Check sheet for the modelled part. Datum: model origin and axes. Units: mm. Give positions to 0.01 mm unless a question says otherwise; leave off trailing zeros. Order: outer loops, then holes, each group sorted by start corner. A loop starts at its lowest first (then second) coordinate and runs counter-clockwise, first axis right, second up.
Item 1: Sectioned sample at A-A on y = 26. Record the boundary of the cut face in (x, z).
Item 2: Sectioned sample at B-B on y = 21.5. Count the separate pieces of the cut face and the enclosed holes in it, and give its area (3 significant figures).
Item 3: Material ranges on line 1 along Y through (x, z) = (22.5, 1.5); line 2 along Z through (x, y) = (20.5, 20); line 3 along X through (y, z) = (-3, 3.5), recorded low to high.
Item 4: Gauge pin test, flat ends, axial feed: P1, Ø5, axis at x = -7, z = 54.5, coming from the -Y side; P2, Ø5, axis at x = 13, y = -1, coming from the +Z side; P3, Ø10, axis at x = 26, z = 17.5, coming from the +Y side; P4, Ø5, axis at x = 29.75, z = 2.76, coming from the -Y side. Record the tip position at first contact, or that the pin passes through.
from build123d import *
from build123d.topology import SkipClean

# Parameters (mm, degrees)
BOSS_EXTRUDE1_START       = -4.7
BOSS_EXTRUDE1_DEPTH       = 4.7
BOSS_EXTRUDE2_OUTLINE_R   = 0.75
BOSS_EXTRUDE2_OUTLINE_R_2 = 2.5
BOSS_EXTRUDE2_DEPTH       = 0.3
SKETCH1_9_R               = 3.95
CUT_EXTRUDE2_DEPTH        = 0.7
SKETCH6_R                 = 0.75
SKETCH6_R_2               = 3.95
BOSS_EXTRUDE6_DEPTH       = 6.25
BOSS_EXTRUDE3_START       = 6.25
SKETCH2_R                 = 5.95
SKETCH2_R_2               = 4.2
BOSS_EXTRUDE3_DEPTH       = 16.25
SKETCH4_R                 = 5.95
SKETCH4_R_2               = 4.2
BOSS_EXTRUDE5_DEPTH       = 5
REVOLVE1_ANGLE            = 10
CUT_EXTRUDE3_DEPTH        = 79.445410831
CIRPATTERN1_COUNT         = 11
CIRPATTERN1_ANGLE         = 85
CUT_EXTRUDE4_DEPTH        = 79.445410831
LPATTERN1_COUNT           = 9
LPATTERN1_PITCH           = 3


# Read off the part's stored shape, not the designer's step: Boss-Extrude2
with BuildPart() as part:
    # Sketch1 → Boss-Extrude1 (new body)
    with BuildSketch(Plane.XZ.offset(-23.543068193).offset(BOSS_EXTRUDE1_START)):
        with BuildLine():
            Line((-0.472592015, 60.640230135), (-2.578285997, 64.210446846))
            ThreePointArc((-2.578285997, 64.210446846), (-11.633365316, 40.543634759), (0.19757138, 18.135123145))
            Line((0.19757138, 18.135123145), (26.104084692, -1.947430003))
            ThreePointArc((26.104084692, -1.947430003), (34.902992649, -0.218708783), (31.996731648, 8.264386483))
            Line((31.996731648, 8.264386483), (8.919209653, 17.677874535))
            ThreePointArc((8.919209653, 17.677874535), (-7.073200942, 36.689574632), (-0.472592015, 60.640230135))
        make_face()
        with BuildLine():
            ThreePointArc((14.223692018, 9.302922077), (13.639231125, 12.051374585), (16.311289521, 12.920678706))
            Line((16.311289521, 12.920678706), (30.419933466, 6.647779521))
            ThreePointArc((30.419933466, 6.647779521), (32.770289273, 5.300105007), (33.699453705, 2.75509961))
            ThreePointArc((33.699453705, 2.75509961), (31.093930231, -0.959046708), (26.714702885, 0.226703387))
            Line((26.714702885, 0.226703387), (14.223692018, 9.302922077))
        make_face(mode=Mode.SUBTRACT)
    extrude(amount=BOSS_EXTRUDE1_DEPTH)

    # Boss-Extrude2 outline → Boss-Extrude2 (add)
    with BuildSketch(Plane.XZ.offset(-23.543068193)):
        with BuildLine():
            Line((-0.472592015, 60.640230135), (-2.578285997, 64.210446846))
            ThreePointArc((-2.578285997, 64.210446846), (-11.633365316, 40.543634759), (0.19757138, 18.135123145))
            Line((0.19757138, 18.135123145), (26.104084692, -1.947430003))
            ThreePointArc((26.104084692, -1.947430003), (34.902992649, -0.218708783), (31.996731648, 8.264386483))
            Line((31.996731648, 8.264386483), (8.919209653, 17.677874535))
            ThreePointArc((8.919209653, 17.677874535), (-7.073200942, 36.689574632), (-0.472592015, 60.640230135))
        make_face()
        with Locations((15.025056724, 11.251695017)):
            Circle(BOSS_EXTRUDE2_OUTLINE_R, mode=Mode.SUBTRACT)
        with Locations((16.757338721, 10.252095558)):
            Circle(BOSS_EXTRUDE2_OUTLINE_R, mode=Mode.SUBTRACT)
        with Locations((18.489620719, 9.252496098)):
            Circle(BOSS_EXTRUDE2_OUTLINE_R, mode=Mode.SUBTRACT)
        with Locations((20.221902717, 8.252896638)):
            Circle(BOSS_EXTRUDE2_OUTLINE_R, mode=Mode.SUBTRACT)
        with Locations((21.954184715, 7.253297178)):
            Circle(BOSS_EXTRUDE2_OUTLINE_R, mode=Mode.SUBTRACT)
        with Locations((23.686466713, 6.253697719)):
            Circle(BOSS_EXTRUDE2_OUTLINE_R, mode=Mode.SUBTRACT)
        with Locations((29.749453705, 2.75509961)):
            Circle(BOSS_EXTRUDE2_OUTLINE_R_2, mode=Mode.SUBTRACT)
        with Locations((25.418748711, 5.254098259)):
            Circle(BOSS_EXTRUDE2_OUTLINE_R, mode=Mode.SUBTRACT)
    extrude(amount=BOSS_EXTRUDE2_DEPTH)

    # Sketch1<9> → Cut-Extrude2 (cut)
    with SkipClean():  # the faces are left unmerged after this step: merging them gives an invalid solid
        with BuildSketch(Plane.XZ.offset(-23.543068193)):
            with Locations(Location((29.749453705, 2.75509961, 0), (0, 0, 270))):
                Circle(SKETCH1_9_R)
        extrude(amount=CUT_EXTRUDE2_DEPTH, mode=Mode.SUBTRACT)

    # Sketch6 → Boss-Extrude6 (add)
    with SkipClean():  # the faces are left unmerged after this step: merging them gives an invalid solid
        with BuildSketch(Plane.XZ.offset(-23.243068193)):
            with BuildLine():
                Line((31.996731648, 8.264386483), (13.649275404, 15.748446521))
                ThreePointArc((13.649275404, 15.748446521), (9.622827675, 14.369008044), (10.443354312, 10.192661811))
                Line((10.443354312, 10.192661811), (26.104084692, -1.947430003))
                ThreePointArc((26.104084692, -1.947430003), (34.902992649, -0.218708783), (31.996731648, 8.264386483))
            make_face()
            with Locations((15.025056724, 11.251695017)):
                Circle(SKETCH6_R, mode=Mode.SUBTRACT)
            with Locations((16.757338721, 10.252095558)):
                Circle(SKETCH6_R, mode=Mode.SUBTRACT)
            with Locations((18.489620719, 9.252496098)):
                Circle(SKETCH6_R, mode=Mode.SUBTRACT)
            with Locations((20.221902717, 8.252896638)):
                Circle(SKETCH6_R, mode=Mode.SUBTRACT)
            with Locations((21.954184715, 7.253297178)):
                Circle(SKETCH6_R, mode=Mode.SUBTRACT)
            with Locations((23.686466713, 6.253697719)):
                Circle(SKETCH6_R, mode=Mode.SUBTRACT)
            with Locations((29.749453705, 2.75509961)):
                Circle(SKETCH6_R_2, mode=Mode.SUBTRACT)
            with Locations((25.418748711, 5.254098259)):
                Circle(SKETCH6_R, mode=Mode.SUBTRACT)
        extrude(amount=BOSS_EXTRUDE6_DEPTH)

    # Sketch2 → Boss-Extrude3 (add)
    with SkipClean():  # the faces are left unmerged after this step: merging them gives an invalid solid
        with BuildSketch(Plane.XZ.offset(-23.243068193).offset(BOSS_EXTRUDE3_START)):
            with Locations(Location((29.749453705, 2.75509961, 0), (0, 0, 232.217400312))):
                Circle(SKETCH2_R)
            with Locations((29.749453705, 2.75509961)):
                Circle(SKETCH2_R_2, mode=Mode.SUBTRACT)
        extrude(amount=BOSS_EXTRUDE3_DEPTH)

    # Sketch4 → Boss-Extrude5 (add)
    # profile 1 of 2: a face of its own
    with SkipClean():  # the faces are left unmerged after this step: merging them gives an invalid solid
        with BuildSketch(Plane.XZ.offset(-0.743068193)):
            with Locations(Location((29.749453705, 2.75509961, 0), (0, 0, 232.217400312))):
                Circle(SKETCH4_R)
            with Locations((29.749453705, 2.75509961)):
                Circle(SKETCH4_R_2, mode=Mode.SUBTRACT)
        # profile 2 of 2: a face of its own
        with BuildSketch(Plane.XZ.offset(-0.743068193)):
            with BuildLine():
                Line((33.215886618, 7.59104242), (7.347230343, 26.133850933))
                ThreePointArc((7.347230343, 26.133850933), (-0.783193574, 39.446224983), (3.120108256, 54.548785387))
                Line((3.120108256, 54.548785387), (0.957208419, 58.215994967))
                ThreePointArc((0.957208419, 58.215994967), (-5.00089426, 42.390828737), (0.954956103, 26.564814703))
                Line((0.954956103, 26.564814703), (25.27600829, -1.168009631))
                ThreePointArc((25.27600829, -1.168009631), (25.34107909, 6.751189354), (33.215886618, 7.59104242))
            make_face()
        extrude(amount=BOSS_EXTRUDE5_DEPTH)

    # Sketch5 → Cut-Revolve1 (revolve, cut)
    with SkipClean():  # the faces are left unmerged after this step: merging them gives an invalid solid
        with BuildSketch(Plane(origin=(7.392091837, 0, 44.324832913), x_dir=(-0.9863772479069666, 0, 0.1644990115820723), z_dir=(-0.1644990115820723, 1.1589156336199524e-15, -0.9863772479069666))):
            with BuildLine():
                ThreePointArc((16.732682915, 18.243068193), (8.385226178, 38.395611457), (-11.767317085, 46.743068193))
                Line((-11.767317085, 46.743068193), (-11.767317085, -10.256931807))
                ThreePointArc((-11.767317085, -10.256931807), (8.385226178, -1.909475071), (16.732682915, 18.243068193))
            make_face()
            with BuildLine():
                Line((-11.767317085, -10.256931807), (-11.767317085, 46.743068193))
                ThreePointArc((-11.767317085, 46.743068193), (-40.267317085, 18.243068193), (-11.767317085, -10.256931807))
            make_face()
        revolve(axis=Axis((18.999105679, 46.743068193, 42.389120883), (0, -1, 0)), mode=Mode.SUBTRACT)

    # Sketch9 → Revolve1 (revolve)
    with SkipClean():  # the faces are left unmerged after this step: merging them gives an invalid solid
        with BuildSketch(Plane(origin=(71.492081558, 0, 33.634820573), x_dir=(0.9863772479069666, 0, -0.1644990115820723), z_dir=(0.1644990115820723, -1.1589156336199524e-15, 0.9863772479069666))):
            with BuildLine():
                Line((-81.275926524, 23.243068193), (-83.905963121, 23.243068193))
                ThreePointArc((-83.905963121, 23.243068193), (-82.209941974, 9.092277505), (-77.21795083, -4.256931807))
                Line((-77.21795083, -4.256931807), (-77.21795083, 0.743068193))
                Line((-77.21795083, 0.743068193), (-75.712394589, 0.743068193))
                ThreePointArc((-75.712394589, 0.743068193), (-80.884704852, 11.401962881), (-81.275926524, 23.243068193))
            make_face()
        revolve(axis=Axis((18.999105679, 28.243068193, 42.389120883), (0, -1, 0)), revolution_arc=REVOLVE1_ANGLE)

    # Sketch11 → Cut-Extrude3 (cut, through all)
    with SkipClean():  # the faces are left unmerged after this step: merging them gives an invalid solid
        with BuildSketch(Plane(origin=(0, 0.743068193, 0), x_dir=(1, 0, 0), z_dir=(0, 1, 0))):
            with BuildLine():
                Line((2.532163802, -53.739884083), (1.289632269, -53.675154355))
                ThreePointArc((1.289632269, -53.675154355), (1.137086791, -53.432140455), (0.987875796, -53.187065043))
                Line((0.987875796, -53.187065043), (1.485316335, -52.046614493))
                ThreePointArc((1.485316335, -52.046614493), (1.987659119, -52.90628238), (2.532163802, -53.739884083))
            make_face()
        cut_extrude3 = extrude(amount=-CUT_EXTRUDE3_DEPTH, mode=Mode.SUBTRACT)

    # CirPattern1: Cut-Extrude3 ×11 about axis
    with SkipClean():  # the faces are left unmerged after this step: merging them gives an invalid solid
        cirpattern1_axis = Axis((18.999105679, 0, 42.389120883), (0, -1, 0))
        for i in range(1, CIRPATTERN1_COUNT):
            add(cut_extrude3.rotate(cirpattern1_axis, i * CIRPATTERN1_ANGLE / (CIRPATTERN1_COUNT - 1)), mode=Mode.SUBTRACT)

    # Sketch13 → Cut-Extrude4 (cut, through all)
    with SkipClean():  # the faces are left unmerged after this step: merging them gives an invalid solid
        with BuildSketch(Plane(origin=(0, 0.743068193, 0), x_dir=(1, 0, 0), z_dir=(0, 1, 0))):
            with BuildLine():
                Line((8.653671949, -25.197385727), (8.63358527, -23.953331438))
                ThreePointArc((8.63358527, -23.953331438), (8.865639921, -23.78458157), (9.099978501, -23.619017963))
                Line((9.099978501, -23.619017963), (10.271673933, -24.037592166))
                Line((10.271673933, -24.037592166), (8.653671949, -25.197385727))
            make_face()
        cut_extrude4 = extrude(amount=-CUT_EXTRUDE4_DEPTH, mode=Mode.SUBTRACT)

    # LPattern1: Cut-Extrude4 ×9
    with SkipClean():  # the faces are left unmerged after this step: merging them gives an invalid solid
        with Locations(*[Vector(0.8127634975154758, 0, -0.5825937667933044) * (i * LPATTERN1_PITCH) for i in range(1, LPATTERN1_COUNT)]):
            add(cut_extrude4, mode=Mode.SUBTRACT)


solid = part.part
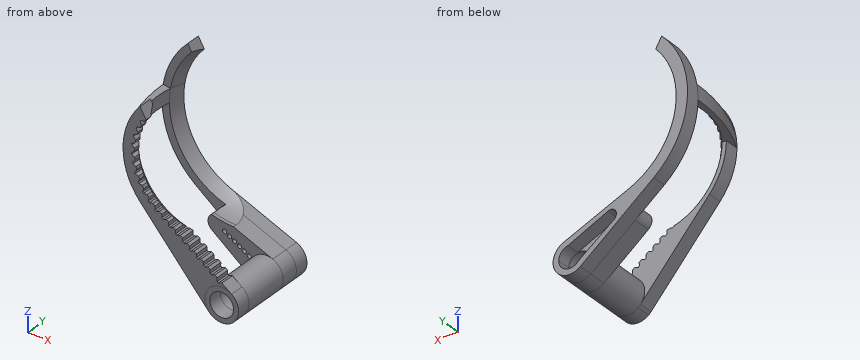
Report:
1. outline: (-2.58, 64.21) arc R30.69 ccw to (0.2, 18.14) - (26.1, -1.95) arc R5.95 ccw (long way) to (32, 8.26) - (14.76, 15.29) arc R27.42 cw to (-0.86, 61.3) - close; hole (14.22, 9.3) - (26.71, 0.23) arc R3.95 ccw (long way) to (30.42, 6.65) - (16.31, 12.92) arc R2.1 ccw to start
2. separate pieces: 2
2. enclosed holes: 8
2. area: 203 mm2
3. line 1: y = 16.99 to 28.24
3. line 2: z = 2.4 to 7.56, 8.95 to 12.95
3. line 3: x = 21.18 to 25.62, 33.88 to 35.65
4. P1: stops at y = 23.24
4. P2: stops at z = 23.81
4. P3: stops at y = 0.74
4. P4: passes through
